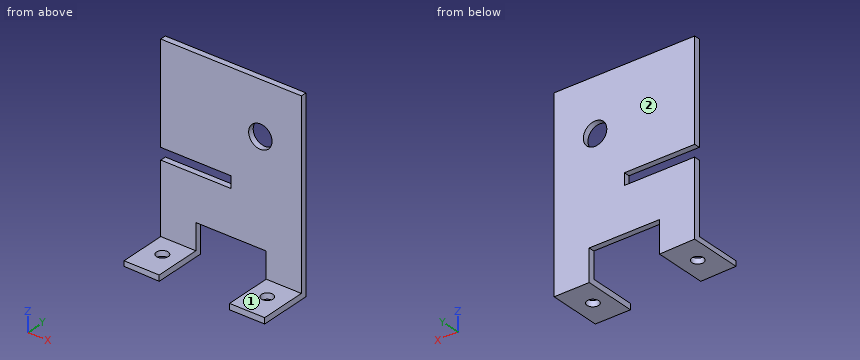
from build123d import *

# Parameters (mm, degrees)
F0_R     = 12.7
F1_DEPTH = 6.35
F2_W     = 38.1
F2_H     = 6.35
F3_DEPTH = 50.8
F4_R     = 6.35
F5_DEPTH = 25.4


with BuildPart() as f1:
    # F0 (on Front) → F1 (new body)
    with BuildSketch(Plane.XZ):
        Polygon((85.480769, 127.986667), (-66.919231, 127.986667), (-66.919231, 20.036667), (9.280769, 20.036667), (9.280769, 7.336667), (-66.919231, 7.336667), (-66.919231, -74.401039), (-28.819231, -75.213333), (-28.819231, -40.757814), (47.380769, -40.757814), (47.380769, -75.213333), (85.480769, -75.213333), align=None)
        with Locations((41.030769, 70.836667)):
            Circle(F0_R, mode=Mode.SUBTRACT)
    extrude(amount=F1_DEPTH)

    # F2 (on face) → F3 (join)
    with BuildSketch(Plane.XZ.offset(6.35)):
        Polygon((-28.819231, -68.863333), (-66.919231, -68.863333), (-66.919231, -74.401039), (-28.819231, -75.213333), align=None)
        with Locations((66.430769, -72.038333)):
            Rectangle(F2_W, F2_H)
    extrude(amount=F3_DEPTH)

    # F4 (on face) → F5 (cut)
    with BuildSketch(Plane(origin=(-1.615918, 0, -75.79331), x_dir=(0.999773, 0, -0.021315), z_dir=(-0.021315, 0, -0.999773))):
        with Locations((-46.263823, 28.575)):
            Circle(F4_R)
        with Locations((67.389801, 28.575)):
            Circle(F4_R)
    extrude(amount=-F5_DEPTH, mode=Mode.SUBTRACT)


solid = f1.part
Model file for the job. Use its own axes, mm. Face numbers are marked on the shaded views. A direction names the side the tool comes from. Give positions to 0.01 mm unless a question says otherwise; leave off trailing zeros. Loops run counter-clockwise (first coordinate to the right, second up) from the corner with the lowest first, then second, coordinate; pieces in that order, holes last.
Item 1: Drill centre lines: line 1 along Y through (x, z) = (16.5, -11); line 2 along Z through (x, y) = (74.5, -37); line 3 along Z through (x, y) = (-60, -34.5). Where is each one in solid material? Low to high.
Check values:
line 1: y = -6.35 to 0
line 2: z = -75.21 to -68.86
line 3: z = -74.55 to -68.86
Item 2: Drop flat-ended pins along their axis: P1, Ø23, axis at x = 41.03, z = 70.84, coming from the -Y side; P2, Ø11.5, axis at x = -44.5, y = -20.5, coming from the +Z side; P3, Ø5, axis at y = -4.5, z = 14, coming from the -X side; P4, Ø7, axis at x = 17.5, y = -4.5, coming from the -Z side. Give the stop position or say it passes through.
Check values:
P1: passes through
P2: stops at z = -68.86
P3: stops at x = 9.28
P4: stops at z = -40.76
Item 3: Slice it at B-B (y = -46.5). Write the cut outline in (x, z).
Check values:
outline: (-66.92, -74.4) - (-28.82, -75.21) - (-28.82, -68.86) - (-66.92, -68.86) - close; (47.38, -75.21) - (85.48, -75.21) - (85.48, -68.86) - (47.38, -68.86) - close
Item 4: Slice it at A-A (x = -15.5). Write the cut outline in (y, z).
Check values:
outline: (-6.35, -40.76) - (0, -40.76) - (0, 7.34) - (-6.35, 7.34) - close; (-6.35, 20.04) - (0, 20.04) - (0, 127.99) - (-6.35, 127.99) - close
Item 5: Which spindle directions (+Z, -Z, +X, -X, +Y, -Y) get a long thin tool onto all of the face, cutting with end or side? Do the marked faces 1 and 2. Say none if no direction does.
Check values:
face 1: +Z, +X, -X, -Y
face 2: +Z, -Z, +X, -X, +Y
Item 6: Slice it at C-C (z = -3.5). Write the cut outline in (x, y), plus the area to 3 significant figures.
Check values:
outline: (-66.92, -6.35) - (85.48, -6.35) - (85.48, 0) - (-66.92, 0) - close
area: 968 mm2
